Build history of the part. All positions in model axes, mm. A direction names the side the tool comes from. Give positions to 0.01 mm unless a question says otherwise; leave off trailing zeros. Loops run counter-clockwise (first coordinate to the right, second up) from the corner with the lowest first, then second, coordinate; pieces in that order, holes last.
1) 3-axis set-ups, long thin cutter, end or side, ignore diameter. For faces 5 (the flat face through (26, 16, 3)), 6 (the flat face through (0, 14, 3)), 7 (the flat face through (-26, 16, 3)), 8 (the flat face through (23, 2, 15)), 9 (the flat face through (2, 25, 7)): which of +Z, -Z, +X, -X, +Y, -Y reach the whole face in a straight line?
2) Band-saw the part on A-A on x = -31. List the corners of the cut face in (y, z).
3) Band-saw the part on C-C on x = 0. List the corners of the cut face in (y, z).
4) Band-saw the part on B-B on y = 14. List the corners of the cut face in (x, z).
5) Two-plate mould, pull along Y, no slides. Class faces 1 (the flat face through (-0.3, 3.5, 7.8)), 2 (the cylindrical face through (25.43, 27.4, 3.55)), 3 (the cylindrical face through (-5.17, 16.4, 1.52)), 4 (the cylindrical face through (-35.4, 3.04, 0.57)): +Y half, -Y half, draft (parallel to the pull), parting line (faces both ways), or undercut.
6) Flat gauge pins, fed straight in: P1, Ø10.5, axis at x = 0, y = 9, coming from the +Z side; P2, Ø4, axis at x = 0.5, y = 1, coming from the +Z side; P3, Ø3, axis at y = 19, z = 4, coming from the -X side. Where does each tip first touch, or does it go through?
7) Band-saw the part on D-D on x = -12.8. List the corners of the cut face in (y, z).
8) Wall check: line 1 (X direction, y = 2.2, z = 7.5); line 2 (Y direction, x = -12.8, z = 0.75); line 3 (X direction, y = 4.25, z = 13). Give the ranges that are in metal, low to high.
```python
from build123d import *

# Parameters (mm, degrees)
BOSS_EXTRU_1_DEPTH      = 15
ESQUISSE2_W             = 46
ESQUISSE2_H             = 21
ENL_V_MAT_EXTRU_1_DEPTH = 12
ESQUISSE4_R             = 8
ENL_V_MAT_EXTRU_2_DEPTH = 3
ENL_V_MAT_EXTRU_3_REACH = 50.01
ESQUISSE5_W             = 12
ESQUISSE5_H             = 7
CONG_1_R                = 2
D_GAGEMENT_M31_D        = 3.4
ENL_V_MAT_EXTRU_4_REACH = 71.663
ESQUISSE10_W            = 8
ESQUISSE10_H            = 25


with BuildPart() as part:
    # Esquisse1 → Boss.-Extru.1 (new body)
    with BuildSketch(Plane.XY):
        Polygon((36, 0), (-36, 0), (-36, 6), (-26, 6), (-26, 28), (26, 28), (26, 6), (36, 6), align=None)
    extrude(amount=BOSS_EXTRU_1_DEPTH)

    # Esquisse2 → Enlèv. mat.-Extru.1 (cut)
    with BuildSketch(Plane.XY.offset(15)):
        with Locations((0, 14)):
            Rectangle(ESQUISSE2_W, ESQUISSE2_H)
    extrude(amount=-ENL_V_MAT_EXTRU_1_DEPTH, mode=Mode.SUBTRACT)

    # Esquisse4 → Enlèv. mat.-Extru.2 (cut)
    with BuildSketch(Plane.XY.offset(3)):
        with Locations((-12.8, 14)):
            Circle(ESQUISSE4_R)
        with Locations((12.8, 14)):
            Circle(ESQUISSE4_R)
    extrude(amount=-ENL_V_MAT_EXTRU_2_DEPTH, mode=Mode.SUBTRACT)

    # Enlèv. mat.-Extru.3: up to this face of the body (flat: up to its plane)
    enl_v_mat_extru_3_end = Plane(part.part.faces().sort_by_distance((0, 28, 7.5))[0])
    # Esquisse5 → Enlèv. mat.-Extru.3 (cut, up to the picked face)
    with BuildSketch(Plane.XZ, mode=Mode.PRIVATE) as enl_v_mat_extru_3_sk1:
        with Locations((0, 11.5)):
            Rectangle(ESQUISSE5_W, ESQUISSE5_H)
    enl_v_mat_extru_3_tool1 = split(extrude(enl_v_mat_extru_3_sk1.sketch, amount=-ENL_V_MAT_EXTRU_3_REACH, mode=Mode.PRIVATE), bisect_by=enl_v_mat_extru_3_end, keep=Keep.BOTH, mode=Mode.PRIVATE)
    add(enl_v_mat_extru_3_tool1.solids().sort_by(Axis((0, 0, 11.5), (0, 1, 0)))[0], mode=Mode.SUBTRACT)

    # Congé1
    cong_1_edges = [part.edges().sort_by_distance(p)[0] for p in [
        (36, 3, 0),
        (-36, 3, 0),
        (36, 3, 15),
        (-26, 28, 7.5),
        (26, 28, 7.5),
        (-36, 3, 15),
    ]]
    fillet(cong_1_edges, radius=CONG_1_R)

    # Dégagement M31 (through all)
    with Locations(Plane(origin=(0, 6, 0), x_dir=(1, 0, 0), z_dir=(0, 1, 0))):
        with Locations((-31, -7.5), (31, -7.5)):
            Hole(D_GAGEMENT_M31_D / 2)

    # Enlèv. mat.-Extru.4: up to this face of the body (flat: up to its plane)
    enl_v_mat_extru_4_end = Plane(part.part.faces().sort_by_distance((-26, 16, 7.5))[0])
    # Esquisse10 → Enlèv. mat.-Extru.4 (cut, up to the picked face)
    with BuildSketch(Plane(origin=(26, 0, 0), x_dir=(0, 0, -1), z_dir=(1, 0, 0)), mode=Mode.PRIVATE) as enl_v_mat_extru_4_sk1:
        with Locations((-11, 18.5)):
            Rectangle(ESQUISSE10_W, ESQUISSE10_H)
    enl_v_mat_extru_4_tool1 = split(extrude(enl_v_mat_extru_4_sk1.sketch, amount=-ENL_V_MAT_EXTRU_4_REACH, mode=Mode.PRIVATE), bisect_by=enl_v_mat_extru_4_end, keep=Keep.BOTH, mode=Mode.PRIVATE)
    add(enl_v_mat_extru_4_tool1.solids().sort_by(Axis((26, 18.5, 11), (-1, 0, 0)))[0], mode=Mode.SUBTRACT)


solid = part.part
```
Findings below:
1. face 5: +Z, -Z, +X, +Y
1. face 6: +Z
1. face 7: +Z, -Z, -X, +Y
1. face 8: +Z, +X, -X, +Y, -Y
1. face 9: +Z, +X, -X, +Y
2. outline: (0, 0) - (6, 0) - (6, 5.8) - (0, 5.8) - close; (0, 9.2) - (6, 9.2) - (6, 15) - (0, 15) - close
3. outline: (0, 0) - (28, 0) - (28, 7) - (24.5, 7) - (24.5, 3) - (3.5, 3) - (3.5, 8) - (0, 8) - close
4. outline: (-26, 0) - (-20.8, 0) - (-20.8, 3) - (-23, 3) - (-23, 7) - (-26, 7) - close; (-4.8, 0) - (4.8, 0) - (4.8, 3) - (-4.8, 3) - close; (20.8, 0) - (26, 0) - (26, 7) - (23, 7) - (23, 3) - (20.8, 3) - close
5. face 1: undercut
5. face 2: +Y half
5. face 3: undercut
5. face 4: draft
6. P1: stops at z = 3
6. P2: stops at z = 8
6. P3: stops at x = -26
7. outline: (0, 0) - (6, 0) - (6, 3) - (3.5, 3) - (3.5, 15) - (0, 15) - close; (22, 0) - (28, 0) - (28, 7) - (24.5, 7) - (24.5, 3) - (22, 3) - close
8. line 1: x = -36 to -32.7, -29.3 to 29.3, 32.7 to 36
8. line 2: y = 0 to 6, 22 to 28
8. line 3: x = -36 to -23, 23 to 36
